Geometry: see drawing. Coordinates: mm, zero at the bounding-box minimum. Give positions to 0.01 mm unless a question says otherwise; leave off trailing zeros. Order: outer loops, then holes, each group sorted by start corner. A loop starts at its lowest first (then second) coordinate and runs counter-clockwise, first axis right, second up. Notation, with made-up numbers: (45, 31.25) - (69, 31.25) arc R29 cw to (69, 70.25) - close; hole circle Ø5 at (1.25, -5). An arc over 180 degrees is marked (long way). One line per item, written item: value.
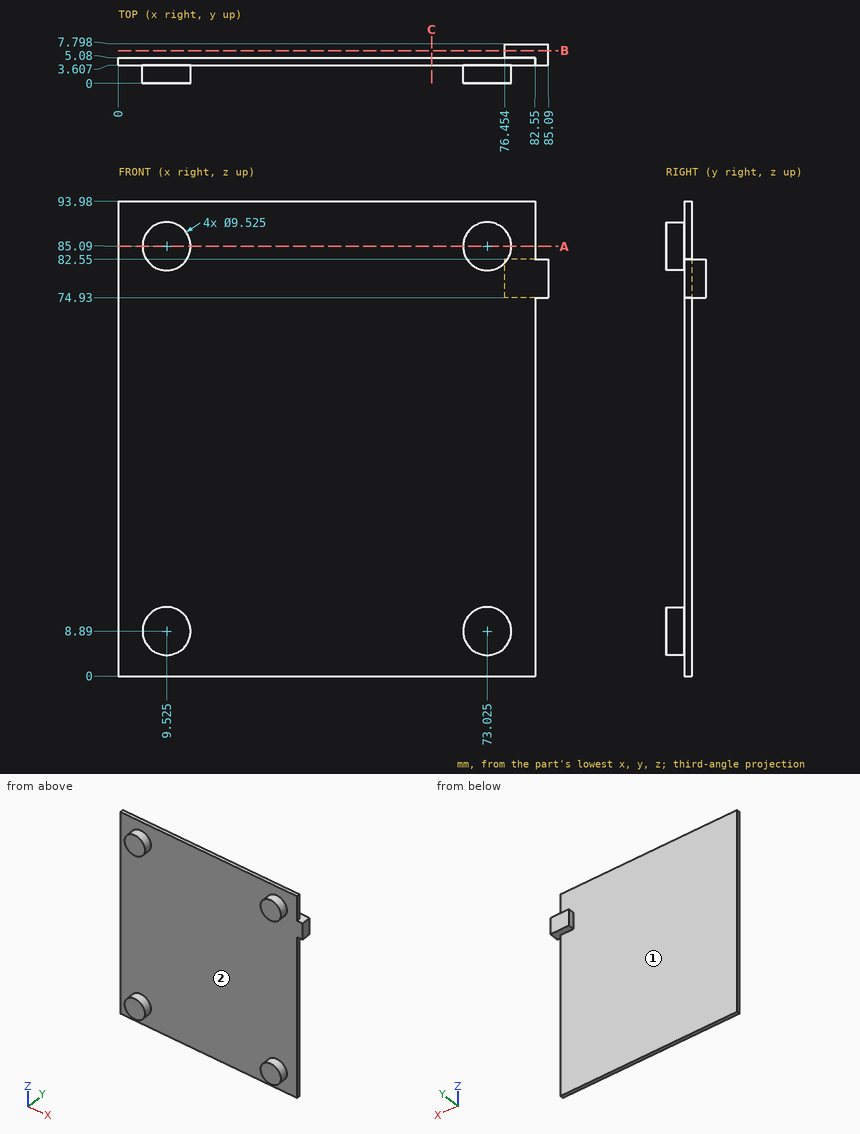
1) Material intervals for line 1 along X through (y, z) = (3, 85); line 2 along Y through (x, z) = (48.5, 39); line 3 along Y through (x, z) = (13, 11.5), sorted ascending.
Answers below:
line 1: 4.76 to 14.29, 68.26 to 77.79
line 2: 3.61 to 5.08
line 3: 0 to 5.08
2) Section C-C, the plane x = 62. Return loops of the section in (y, z).
Answers below:
outline: (3.61, 0) - (5.08, 0) - (5.08, 93.98) - (3.61, 93.98) - close
3) Section A-A, the plane z = 85.09. Return loops of the section in (x, y).
Answers below:
outline: (0, 3.61) - (4.76, 3.61) - (4.76, 0) - (14.29, 0) - (14.29, 3.61) - (68.26, 3.61) - (68.26, 0) - (77.79, 0) - (77.79, 3.61) - (82.55, 3.61) - (82.55, 5.08) - (0, 5.08) - close
4) First-contact query: pin 1 (6 mm diameter, centred on x = 65.5, z = 40.5, fed in from -Y); pin 2 (0.8 mm diameter, centred on y = 6, z = 77.5, fed in from -X); pin 3 (1 mm diameter, centred on x = 34, z = 22.5, fed in from +Y). Flat tips, straight axial feed; report the tip coordinate or a pass-through.
Answers below:
pin 1: y = 3.61
pin 2: x = 76.45
pin 3: y = 5.08
5) Section B-B, the plane y = 6.5. Return loops of the section in (x, z).
Answers below:
outline: (76.45, 74.93) - (85.09, 74.93) - (85.09, 82.55) - (76.45, 82.55) - close
6) Mould query, pull axis Z, two halves, no side actions, for the marked faces 1 and 2. Classes: released by +Z, released by -Z, zero draft, split by the parting line, or undercut.
Answers below:
face 1: zero draft
face 2: undercut
